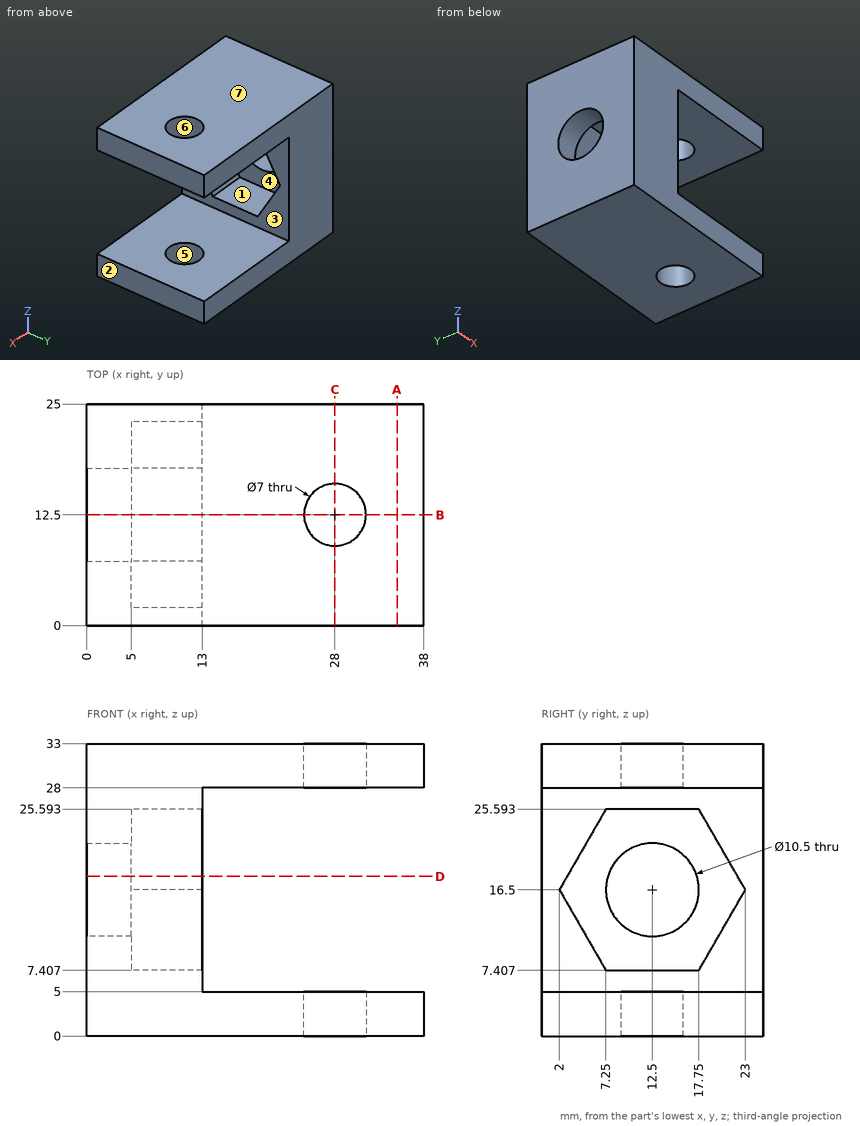
Here's the drawing with two shaded views (mm, measured from the low corner). I have some questions. A direction names the side the tool comes from. Coordinates: 2 decimals unless noted, no trailing zeros. Write each loop counter-clockwise with the first axis right and the second up, starting at its lowest first coordinate (ties: lowest second). Pieces come first, ordered by that corner, then holes. Notation, with made-up numbers: (26.25, 74) -> (48.25, 74) arc R16 cw to (48.25, 96) -> close; hole circle Ø3 at (10.25, 42). An arc over 180 degrees is marked (long way). One line per question, with ' | ' between items. Start each with the question number.
1. Please list where these lines run through material, in increasing order: line 1 along Y through (x, z) = (28, 3); line 2 along Z through (x, y) = (19, 19.25); line 3 along Y through (x, z) = (7.5, 16.5).
2. Will these pins go through, and if not, where does the flat tip stop? P1, Ø2.5, axis at x = 7, y = 12.5, coming from the -Z side; P2, Ø5.5, axis at x = 28, y = 12.5, coming from the +Z side; P3, Ø4, axis at y = 8.5, z = 21, coming from the +X side; P4, Ø9, axis at y = 8.5, z = 12.5, coming from the +X side.
3. Thinking about a two-plate mould opening in X: for the marked faces 4, 5, 6 and 7, which applies, pulls with the +X half, pulls with the -X half, needs draft (parallel to the pull), parting line crosses it, or undercut?
4. If we section it at A-A (x = 35): Please give me the cut outline in (y, z).
5. For the marked faces 1, 2 and 3, which set-ups out of +Z, -Z, +X, -X, +Y, -Y let a thin tool reach every point of the face, with its end or its side?
6. If we section it at B-B (y = 12.5): Please give me the cut outline in (x, z), and give its area (3 significant figures).
7. If we section it at C-C (x = 28): Please give me the cut outline in (y, z), and give its area (3 significant figures).
8. If we section it at D-D (z = 18): Please give me the cut outline in (x, y), and give its area (3 significant figures).
Return value:
1) line 1: y = 0 to 9, 16 to 25 | line 2: z = 0 to 5, 28 to 33 | line 3: y = 0 to 2, 23 to 25
2) P1: stops at z = 0 | P2: passes through | P3: stops at x = 5 | P4: stops at x = 13
3) face 4: pulls with the +X half | face 5: undercut | face 6: undercut | face 7: needs draft
4) outline: (0, 0) -> (25, 0) -> (25, 5) -> (0, 5) -> close; (0, 28) -> (25, 28) -> (25, 33) -> (0, 33) -> close
5) face 1: +X | face 2: +Z, -Z, +X, +Y, -Y | face 3: +X, +Y, -Y
6) outline: (0, 0) -> (24.5, 0) -> (24.5, 5) -> (13, 5) -> (13, 7.41) -> (5, 7.41) -> (5, 11.25) -> (0, 11.25) -> close; (0, 21.75) -> (5, 21.75) -> (5, 25.59) -> (13, 25.59) -> (13, 28) -> (24.5, 28) -> (24.5, 33) -> (0, 33) -> close; (31.5, 0) -> (38, 0) -> (38, 5) -> (31.5, 5) -> close; (31.5, 28) -> (38, 28) -> (38, 33) -> (31.5, 33) -> close | area: 411 mm²
7) outline: (0, 0) -> (9, 0) -> (9, 5) -> (0, 5) -> close; (0, 28) -> (9, 28) -> (9, 33) -> (0, 33) -> close; (16, 0) -> (25, 0) -> (25, 5) -> (16, 5) -> close; (16, 28) -> (25, 28) -> (25, 33) -> (16, 33) -> close | area: 180 mm²
8) outline: (0, 0) -> (13, 0) -> (13, 2.87) -> (5, 2.87) -> (5, 7.47) -> (0, 7.47) -> close; (0, 17.53) -> (5, 17.53) -> (5, 22.13) -> (13, 22.13) -> (13, 25) -> (0, 25) -> close | area: 121 mm²
